CAD build for the part. Positions are in the model's coordinates, mm. A direction names the side the tool comes from. Give positions to 0.01 mm unless a question says otherwise; leave off trailing zeros. Write each loop counter-clockwise with the first axis right and the second up, starting at its lowest first coordinate (ties: lowest second). Pieces come first, ordered by that corner, then holes. Notation, with made-up numbers: (-24, 70) -> (35, 70) arc R12 cw to (35, 88) -> close; hole circle Ø5 at (-9.75, 0.25). An arc over 180 degrees is marked (long way). Use one line per item in the form item = value. Start each with the question number.
from build123d import *

# Parameters (mm, degrees)
SKETCH1_W                        = 55.88
SKETCH1_H                        = 19.685
EXTRUDE1_DEPTH                   = 42.926
SKETCH3_OUTSIDE_W                = 72.512
SKETCH3_OUTSIDE_H                = 36.318
SKETCH3_OUTSIDE_R                = 2.9718
EXTRUDE2_DEPTH                   = 5.334
SKETCH8_W                        = 7.62
SKETCH8_H                        = 19.685
EXTRUDE5_DEPTH                   = 26.289
F_39_0_0995_DIAMETER_HOLE1_D     = 2.5273
F_39_0_0995_DIAMETER_HOLE1_DEPTH = 12.7
F_39_0_0995_DIAMETER_HOLE1_TIP   = 0.759277521
SKETCH13_W                       = 7.62
SKETCH13_H                       = 19.685
EXTRUDE6_DEPTH                   = 6.5278


with BuildPart() as part:
    # Sketch1 → Extrude1 (new body)
    with BuildSketch(Plane.XY):
        Rectangle(SKETCH1_W, SKETCH1_H)
    extrude(amount=EXTRUDE1_DEPTH)

    # Sketch3 outside → Extrude2 (cut)
    with BuildSketch(Plane.XY.offset(42.926)):
        Rectangle(SKETCH3_OUTSIDE_W, SKETCH3_OUTSIDE_H)
        with Locations((-9.398, 0)):
            Circle(SKETCH3_OUTSIDE_R, mode=Mode.SUBTRACT)
    extrude(amount=-EXTRUDE2_DEPTH, mode=Mode.SUBTRACT)

    # Sketch8 → Extrude5 (cut)
    with BuildSketch(Plane(origin=(0, 0, 0), x_dir=(-1, 0, 0), z_dir=(0, 0, -1))):
        with Locations((-24.13, 0)):
            Rectangle(SKETCH8_W, SKETCH8_H)
        with Locations((24.13, 0)):
            Rectangle(SKETCH8_W, SKETCH8_H)
    extrude(amount=-EXTRUDE5_DEPTH, mode=Mode.SUBTRACT)

    # #39 (0.0995) Diameter Hole1
    with Locations(Plane(origin=(-24.765, 4.953, 37.592), x_dir=(1, 0, 0), z_dir=(0, 0, 1))):
        with Locations((0, 0), (0, -9.906), (49.53, 0), (49.53, -9.906)):
            Hole(F_39_0_0995_DIAMETER_HOLE1_D / 2, depth=F_39_0_0995_DIAMETER_HOLE1_DEPTH)
            with Locations((0, 0, -(F_39_0_0995_DIAMETER_HOLE1_DEPTH + F_39_0_0995_DIAMETER_HOLE1_TIP / 2))):  # 118° drill point
                Cone(0, F_39_0_0995_DIAMETER_HOLE1_D / 2, F_39_0_0995_DIAMETER_HOLE1_TIP, mode=Mode.SUBTRACT)

    # Sketch13 → Extrude6 (cut)
    with BuildSketch(Plane.XY.offset(37.592)):
        with Locations((-24.13, 0)):
            Rectangle(SKETCH13_W, SKETCH13_H)
        with Locations((24.13, 0)):
            Rectangle(SKETCH13_W, SKETCH13_H)
    extrude(amount=-EXTRUDE6_DEPTH, mode=Mode.SUBTRACT)


solid = part.part
1) 3-axis set-ups, long thin cutter, end or side, ignore diameter. For faces 1 (the face through (20.32, 0, 34)), 2 (the face through (-20.32, 0, 34)), 3 (the face through (24, 0, 26.289)), 4 (the face through (-6.563, 0.893, 40.296)), 5 (the face through (-24, 0, 26.289)): which of +Z, -Z, +X, -X, +Y, -Y reach the whole face in a straight line?
2) Pin check, flat tips, straight feed: pin 1 (10 mm diameter, centred on y = -4.5, z = 8.5, fed in from +X); pin 2 (8.5 mm diameter, centred on x = 22.5, y = -4, fed in from +Z); pin 3 (2.5 mm diameter, centred on x = 24, y = 1, fed in from -Z). Stop position of each tip, or through.
3) Cut at B-B (x = -11). Give the cut face in (y, z), and give its area (3 significant figures).
4) Cut at C-C (z = 18.5). Give the cut face in (x, y).
5) Two-plate mould, pull along X, no slides. Class faces 6 (the face through (-25.97, 5.33, 28.64)), 7 (the face through (24, 0, 31.064)), 8 (the face through (-27.94, 0, 29)): released by +X, released by -X, zero draft, split by the parting line, or undercut.
6) Cut at A-A (y = 0). Give the cut face in (x, z), and give its area (3 significant figures).
7) Cut at D-D (y = 8). Give the cut face in (x, z), and give its area (3 significant figures).
8) Wall check: line 1 along X through (y, z) = (-5.75, 3.5); line 2 along Z through (x, y) = (19, 4.5); line 3 along Z through (x, y) = (-22.5, 6). Give the ranges that are in metal, low to high. Write a range as from..to.
Final values:
q1.face_1 = +Z, +X, +Y, -Y
q1.face_2 = +Z, -X, +Y, -Y
q1.face_3 = -Z, +X, +Y, -Y
q1.face_4 = +Z
q1.face_5 = -Z, -X, +Y, -Y
q2.pin_1 = 20.32
q2.pin_2 = 37.59
q2.pin_3 = 26.29
q3.outline = (-9.84, 0) -> (9.84, 0) -> (9.84, 37.59) -> (2.5, 37.59) -> (2.5, 42.93) -> (-2.5, 42.93) -> (-2.5, 37.59) -> (-9.84, 37.59) -> close
q3.area = 767 mm^2
q4.outline = (-20.32, -9.84) -> (20.32, -9.84) -> (20.32, 9.84) -> (-20.32, 9.84) -> close
q5.face_6 = undercut
q5.face_7 = zero draft
q5.face_8 = released by -X
q6.outline = (-27.94, 26.29) -> (-20.32, 26.29) -> (-20.32, 0) -> (20.32, 0) -> (20.32, 26.29) -> (27.94, 26.29) -> (27.94, 31.06) -> (20.32, 31.06) -> (20.32, 37.59) -> (-6.43, 37.59) -> (-6.43, 42.93) -> (-12.37, 42.93) -> (-12.37, 37.59) -> (-20.32, 37.59) -> (-20.32, 31.06) -> (-27.94, 31.06) -> close
q6.area = 1,630 mm^2
q7.outline = (-27.94, 26.29) -> (-20.32, 26.29) -> (-20.32, 0) -> (20.32, 0) -> (20.32, 26.29) -> (27.94, 26.29) -> (27.94, 31.06) -> (20.32, 31.06) -> (20.32, 37.59) -> (-20.32, 37.59) -> (-20.32, 31.06) -> (-27.94, 31.06) -> close
q7.area = 1,600 mm^2
q8.line_1 = -20.32..20.32
q8.line_2 = 0..37.59
q8.line_3 = 26.29..31.06
